Geometry check sheet. Reference: the model listing, model coordinates, mm. A direction names the side the tool comes from. Coordinates: 2 decimals unless noted, no trailing zeros. Order: outer loops, then holes, each group sorted by start corner. A loop starts at its lowest first (then second) coordinate and runs counter-clockwise, first axis right, second up. Notation, with made-up numbers: (23, -2) - (61, -2) arc R12 cw to (61, 3) - close; hole circle Ø10 at (28.5, 24.5). An arc over 180 degrees is marked (long way). Put each result on its own line as item: value.
from build123d import *

# Parameters (mm, degrees)
SKETCH1_W                                        = 32
SKETCH1_H                                        = 52
BOSS_EXTRUDE1_DEPTH                              = 9
CUT_EXTRUDE2_DEPTH                               = 58.078892771
F_10_0_10_DIAMETER_HOLE1_D                       = 10
FILLET3_R                                        = 12
CUT_EXTRUDE3_DEPTH                               = 58.078892771
CUT_EXTRUDE3_DEPTH_BACK                          = 58.078892771
M4X0_7_TAPPED_HOLE2_D                            = 2.1
M4X0_7_TAPPED_HOLE2_CBORE_D                      = 3.3
M4X0_7_TAPPED_HOLE2_CBORE_DEPTH                  = 2
CBORE_FOR_M3_HEX_HEAD_MACHINE_SCREW5_D           = 3.2
CBORE_FOR_M3_HEX_HEAD_MACHINE_SCREW5_CBORE_D     = 10.2
CBORE_FOR_M3_HEX_HEAD_MACHINE_SCREW5_CBORE_DEPTH = 1
F_4_1_4_1_DIAMETER_HOLE3_D                       = 4.1
CUT_EXTRUDE4_DEPTH                               = 58.078892771
CUT_EXTRUDE4_DEPTH_BACK                          = 58.078892771


with BuildPart() as part:
    # Sketch1 → Boss-Extrude1 (new body)
    with BuildSketch(Plane(origin=(-2, 0, 0), x_dir=(0, -1, 0), z_dir=(-1, 0, 0))):
        with Locations((-8, 25)):
            Rectangle(SKETCH1_W, SKETCH1_H)
    extrude(amount=-BOSS_EXTRUDE1_DEPTH)

    # Sketch3 → Cut-Extrude2 (cut, through all)
    with BuildSketch(Plane(origin=(7, 0, 0), x_dir=(0, 0, -1), z_dir=(1, 0, 0))):
        Polygon((4, 6.75), (-18, 6.75), (-20, 24), (4, 24), align=None)
    extrude(amount=-CUT_EXTRUDE2_DEPTH, mode=Mode.SUBTRACT)

    # Ø10.0 (10) Diameter Hole1 (through all)
    with Locations(Plane.ZY.offset(2)):
        with Locations((28, 0)):
            Hole(F_10_0_10_DIAMETER_HOLE1_D / 2)

    # Fillet3
    fillet3_edges = [part.edges().sort_by_distance(p)[0] for p in [
        (2.5, -8, 51),
    ]]
    fillet(fillet3_edges, radius=FILLET3_R)

    # Cut-Sweep1: sweep along a path in Sketch22
    with BuildLine(Plane(origin=(-2, 0, 0), x_dir=(0, -1, 0), z_dir=(-1, 0, 0))) as cut_sweep1_path:
        Line((8, 11), (-6.75, 4.890349955))
    # Sketch21 → Cut-Sweep1 (sweep, cut)
    with BuildSketch(Plane.XZ.offset(8)):
        Polygon((7, 7), (5.5, 7), (4, 10), (7, 10), align=None)
        Polygon((1, 10), (-0.5, 7), (-2, 7), (-2, 10), align=None)
    sweep(path=cut_sweep1_path.line, mode=Mode.SUBTRACT)

    # Sketch23 → Cut-Extrude3 (cut, two sides: drawn at the far end of the back side and taken through both)
    with BuildSketch(Plane.ZY.offset(2).offset(-CUT_EXTRUDE3_DEPTH_BACK)):
        Polygon((-1, 6.75), (-1, -8), (7, -8), (0.890349955, 6.75), align=None)
    extrude(amount=CUT_EXTRUDE3_DEPTH + CUT_EXTRUDE3_DEPTH_BACK, mode=Mode.SUBTRACT)

    # M4x0.7 Tapped Hole2 (through all)
    with Locations(Plane(origin=(-2, 13.349760492, 32.849760492), x_dir=(0, 0, -1), z_dir=(-1, 0, 0))):
        with Locations((0, 0), (-12.75, -7.361215932), (-12.75, 7.361215932)):
            CounterBoreHole(M4X0_7_TAPPED_HOLE2_D / 2, M4X0_7_TAPPED_HOLE2_CBORE_D / 2, M4X0_7_TAPPED_HOLE2_CBORE_DEPTH)

    # CBORE for M3 Hex Head Machine Screw5 (through all)
    with Locations(Plane(origin=(7, 13.349760492, 41.349760492), x_dir=(0, 0, 1), z_dir=(1, 0, 0))):
        with Locations((0, 0)):
            CounterBoreHole(CBORE_FOR_M3_HEX_HEAD_MACHINE_SCREW5_D / 2, CBORE_FOR_M3_HEX_HEAD_MACHINE_SCREW5_CBORE_D / 2, CBORE_FOR_M3_HEX_HEAD_MACHINE_SCREW5_CBORE_DEPTH)

    # Ø4.1 (4.1) Diameter Hole3 (through all)
    with Locations(Plane(origin=(-2, 14, 25.510762466), x_dir=(0, 0, -1), z_dir=(-1, 0, 0))):
        with Locations((0, 0)):
            Hole(F_4_1_4_1_DIAMETER_HOLE3_D / 2)

    # Sketch37 → Cut-Extrude4 (cut, two sides: drawn at the far end of the back side and taken through both)
    with BuildSketch(Plane.ZY.offset(2).offset(-CUT_EXTRUDE4_DEPTH_BACK)):
        Polygon((33.300431818, 19.554652238), (41, 24), (20, 24), (19.874101839, 22.914128361), (19.484597361, 19.554652238), align=None)
    extrude(amount=CUT_EXTRUDE4_DEPTH + CUT_EXTRUDE4_DEPTH_BACK, mode=Mode.SUBTRACT)


solid = part.part
Q1. Depth check by flat-ended pin: pin 1 Ø1 at (x, y) = (3, 0.5) entering from -Z; pin 2 Ø5 at (x, y) = (1.5, 9) entering from -Z; pin 3 Ø1.6 at (y, z) = (6, 46) entering from -X. Enter the tip coordinate at first touch or a pass-through.
Answer block:
pin 1: stops at z = 3.27
pin 2: stops at z = 0.89
pin 3: stops at x = 0
Q2. Section check A-A on x = 4.75. Record the boundary of the cut face in (y, z), then the cut area to 3 significant figures.
Answer block:
outline: (-8, 7) - (6.75, 0.89) - (6.75, 2.39) - (-8, 8.5) - close; (-8, 10) - (6.75, 3.89) - (6.75, 18) - (19.55, 19.48) - (19.55, 33.3) - (24, 41) - (24, 51) - (4, 51) arc R12 ccw to (-8, 39) - close; hole circle Ø10 at (0, 28); hole circle Ø2.1 at (5.99, 45.6); hole circle Ø3.2 at (13.35, 41.35); hole circle Ø4.1 at (14, 25.51); hole circle Ø2.1 at (13.35, 32.85); hole circle Ø2.1 at (20.71, 45.6)
area: 1,010 mm^2
Q3. Section check D-D on y = -4.5. Record the boundary of the cut face in (x, z), then the cut area to 3 significant figures.
Answer block:
outline: (-2, 8.55) - (1, 8.55) - (-0.5, 5.55) - (5.5, 5.55) - (4, 8.55) - (7, 8.55) - (7, 25.82) - (-2, 25.82) - close; (-2, 30.18) - (7, 30.18) - (7, 47.47) - (-2, 47.47) - close
area: 325 mm^2
Q4. Thickness scan on L1, parallel to Y at x = 6, z = 15; L2, parallel to X at y = 17, z = 41; L3, parallel to Z at x = 1, y = 14. Record the ranges inside material, lowest first. Write a range as [from, to].
Answer block:
L1: y = [-8, 6.75]
L2: x = [-2, 6]
L3: z = [18.84, 23.46], [27.56, 32.03], [33.67, 39.89], [42.81, 51]
Q5. Section check C-C on x = -1.5. Record the boundary of the cut face in (y, z).
Answer block:
outline: (-8, 10) - (6.75, 3.89) - (6.75, 18) - (19.55, 19.48) - (19.55, 33.3) - (24, 41) - (24, 51) - (4, 51) arc R12 ccw to (-8, 39) - close; hole circle Ø10 at (0, 28); hole circle Ø3.3 at (5.99, 45.6); hole circle Ø3.3 at (13.35, 32.85); hole circle Ø3.2 at (13.35, 41.35); hole circle Ø4.1 at (14, 25.51); hole circle Ø3.3 at (20.71, 45.6)
Q6. Access from +Z, -Z, +X, -X, +Y, -Y to the whole of each face (thin tool, end or side, straight path). Record for faces 4 (the flat face through (2.56, 13.06, 18.73)), 5 (the cylindrical face through (-1.014, 6.621, 44.076)), 6 (the flat face through (5.52, -0.52, 6.9)).
Answer block:
face 4: -Z, +X, -X, +Y
face 5: -X
face 6: +X
Q7. Section check B-B on y = 0. Record the boundary of the cut face in (x, z), then the cut area to 3 significant figures.
Answer block:
outline: (-2, 6.69) - (1, 6.69) - (-0.5, 3.69) - (5.5, 3.69) - (4, 6.69) - (7, 6.69) - (7, 23) - (-2, 23) - close; (-2, 33) - (7, 33) - (7, 50.31) - (-2, 50.31) - close
area: 316 mm^2
Q8. Draft check along Z on faces 1 (the flat face through (2, 14, 51)), 2 (the flat face through (-2, 5, 33)), 3 (the cylindrical face through (3, 0, 33)). Enter one of: pulls with the +Z half, pulls with the -Z half, needs draft (parallel to the pull), parting line crosses it, or undercut.
Answer block:
face 1: pulls with the +Z half
face 2: needs draft
face 3: undercut
